Input: dimensioned drawing with shaded views. Units: mm. Origin: part minimum x, y, z. A direction names the side the tool comes from. Round coordinates to 2 decimals unless told otherwise and drop trailing zeros. Order: outer loops, then holes, each group sorted by start corner. A loop starts at its lowest first (then second) coordinate and runs counter-clockwise, first axis right, second up. Notation, with made-up numbers: M 13,40.5 L 24,40.5 A16 ccw 24,71.5 Z; hole C 15.25,0.25 d7. An arc over 180 degrees is marked long. Answer as CSV lines item,"result". Start each with the question number.
Item 1: Line query: line 1 (X direction, y = 26.5, z = 10.5); line 2 (Z direction, x = 22.5, y = 12); line 3 (Y direction, x = 24, z = 41.5). Output: solid intervals per line, ascending. Write a range as [from, to].
Item 2: Section query C-C on x = 23.5. Return the cut outline in (y, z).
Item 3: Section query B-B on z = 36.5. Return the cut outline in (x, y).
Item 4: Section query A-A on y = 32.5. Return the cut outline in (x, z), plus the area to 3 significant figures.
Item 5: First-contact query: P1, Ø10, axis at x = 18.5, y = 44, coming from the -Z side; P2, Ø11, axis at x = 26, z = 13.5, coming from the -Y side. Flat tips, straight axial feed; report the tip coordinate or a pass-through.
Item 6: Set-up query: the marked faces 1 and 2. Return all of +Z, -Z, +X, -X, +Y, -Y with unobstructed straight access to the full face (end or side cutting, diameter ignored); none if empty.
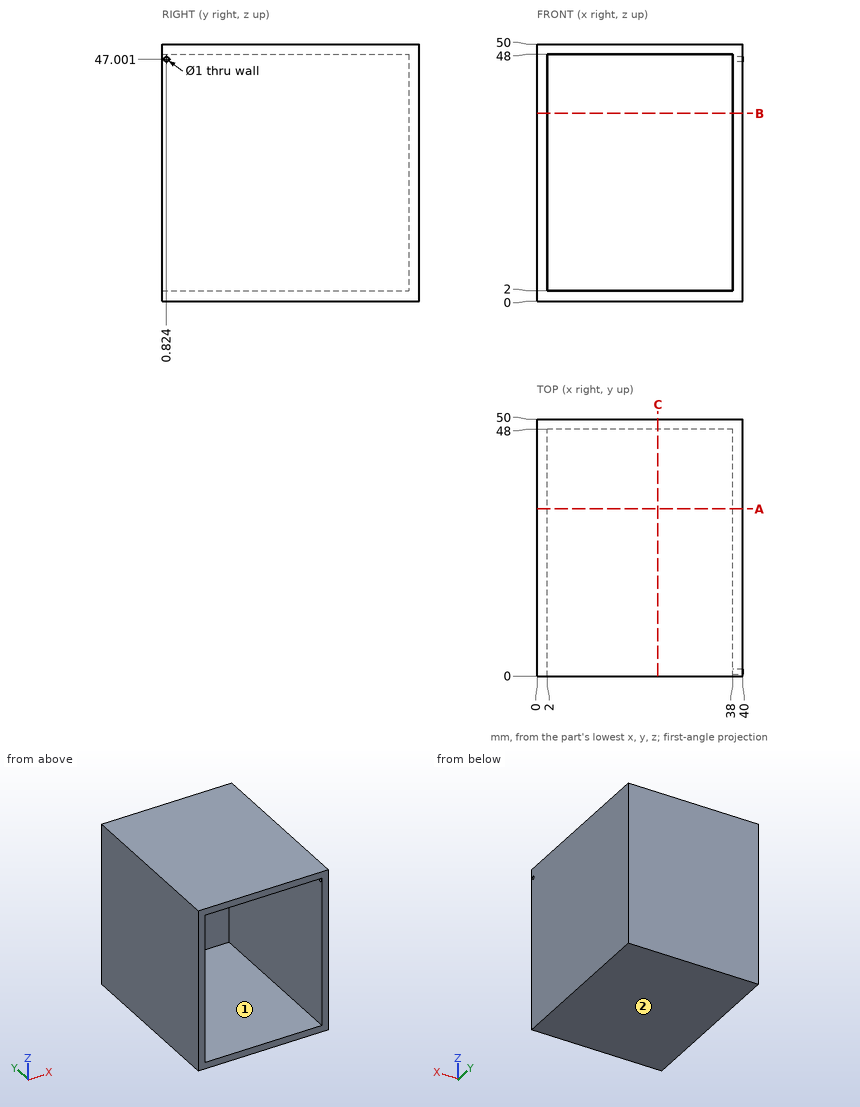
Results:
1,line 1,"[0, 2], [38, 40]"
1,line 2,"[0, 2], [48, 50]"
1,line 3,"[48, 50]"
2,outline,"M 0,0 L 50,0 L 50,50 L 0,50 L 0,48 L 48,48 L 48,2 L 0,2 Z"
3,outline,"M 0,0 L 2,0 L 2,48 L 38,48 L 38,0 L 40,0 L 40,50 L 0,50 Z"
4,outline,"M 0,0 L 40,0 L 40,50 L 0,50 Z; hole M 2,2 L 38,2 L 38,48 L 2,48 Z"
4,area,"344 mm^2"
5,P1,"z = 0"
5,P2,"y = 48"
6,face 1,"-Y"
6,face 2,"-Z, +X, -X, +Y, -Y"
